```python
from build123d import *

# Parameters (mm, degrees)
ESQUISSE1_R             = 1.7
BOSS_EXTRU_1_DEPTH      = 3
ESQUISSE2_R             = 5.2
BOSS_EXTRU_2_DEPTH      = 3
BOSS_EXTRU_2_DEPTH_BACK = 3
ESQUISSE5_W             = 129.390100882
ESQUISSE5_H             = 125.631489025
ENL_V_MAT_EXTRU_2_DEPTH = 1
ESQUISSE6_R             = 1.5
ENL_V_MAT_EXTRU_3_DEPTH = 8
ESQUISSE7_W             = 14.610679854
ESQUISSE7_H             = 62.75
ENL_V_MAT_EXTRU_4_DEPTH = 8
BOSS_EXTRU_3_DEPTH      = 7
BOSS_EXTRU_4_DEPTH      = 7
ESQUISSE11_W            = 143.807333736
ESQUISSE11_H            = 19.954067826
ENL_V_MAT_EXTRU_5_DEPTH = 89
ESQUISSE12_R            = 1.7
ENL_V_MAT_EXTRU_6_DEPTH = 31


with BuildPart() as part:
    # Esquisse1 → Boss.-Extru.1 (new body)
    with BuildSketch(Plane.XY):
        with BuildLine():
            Line((-117.680084405, 66.939310237), (-117.680084405, 59.695120061))
            ThreePointArc((-117.680084405, 59.695120061), (-116.069171702, 55.806032765), (-112.180084405, 54.195120061))
            Line((-112.180084405, 54.195120061), (-105.294175096, 54.195120061))
            ThreePointArc((-105.294175096, 54.195120061), (-101.4050878, 52.584207358), (-99.794175096, 48.695120061))
            Line((-99.794175096, 48.695120061), (-99.794175096, 35.930823665))
            ThreePointArc((-99.794175096, 35.930823665), (-101.4050878, 32.041736368), (-105.294175096, 30.430823665))
            Line((-105.294175096, 30.430823665), (-112.180084405, 30.430823665))
            ThreePointArc((-112.180084405, 30.430823665), (-116.069171702, 28.819910961), (-117.680084405, 24.930823665))
            Line((-117.680084405, 24.930823665), (-117.680084405, 23.910007682))
            ThreePointArc((-117.680084405, 23.910007682), (-116.069171702, 20.020920385), (-112.180084405, 18.410007682))
            Line((-112.180084405, 18.410007682), (-105.294175096, 18.410007682))
            ThreePointArc((-105.294175096, 18.410007682), (-101.4050878, 16.799094979), (-99.794175096, 12.910007682))
            Line((-99.794175096, 12.910007682), (-99.794175096, 1.692208933))
            ThreePointArc((-99.794175096, 1.692208933), (-101.4050878, -2.196878364), (-105.294175096, -3.807791067))
            Line((-105.294175096, -3.807791067), (-113.390601299, -3.807791067))
            ThreePointArc((-113.390601299, -3.807791067), (-117.279688595, -5.418703771), (-118.890601299, -9.307791067))
            Line((-118.890601299, -9.307791067), (-118.890601299, -18.42196685))
            Line((-118.890601299, -18.42196685), (-118.890601299, -32.5606385))
            ThreePointArc((-118.890601299, -32.5606385), (-117.279688595, -36.449725797), (-113.390601299, -38.0606385))
            Line((-113.390601299, -38.0606385), (-52.866544484, -38.0606385))
            ThreePointArc((-52.866544484, -38.0606385), (-48.977457187, -36.449725797), (-47.366544484, -32.5606385))
            Line((-47.366544484, -32.5606385), (-47.366544484, -18.42196685))
            Line((-47.366544484, -18.42196685), (-47.366544484, -9.307791067))
            ThreePointArc((-47.366544484, -9.307791067), (-48.977457187, -5.418703771), (-52.866544484, -3.807791067))
            Line((-52.866544484, -3.807791067), (-77.986378892, -3.807791067))
            ThreePointArc((-77.986378892, -3.807791067), (-81.875466189, -2.196878364), (-83.486378892, 1.692208933))
            Line((-83.486378892, 1.692208933), (-83.486378892, 12.910007682))
            ThreePointArc((-83.486378892, 12.910007682), (-81.875466189, 16.799094979), (-77.986378892, 18.410007682))
            Line((-77.986378892, 18.410007682), (-69.856378892, 18.410007682))
            ThreePointArc((-69.856378892, 18.410007682), (-65.967291596, 20.020920385), (-64.356378892, 23.910007682))
            Line((-64.356378892, 23.910007682), (-64.356378892, 24.930823665))
            ThreePointArc((-64.356378892, 24.930823665), (-65.967291596, 28.819910961), (-69.856378892, 30.430823665))
            Line((-69.856378892, 30.430823665), (-77.986378892, 30.430823665))
            ThreePointArc((-77.986378892, 30.430823665), (-81.875466189, 32.041736368), (-83.486378892, 35.930823665))
            Line((-83.486378892, 35.930823665), (-83.486378892, 55.219310237))
            ThreePointArc((-83.486378892, 55.219310237), (-81.875466189, 59.108397534), (-77.986378892, 60.719310237))
            Line((-77.986378892, 60.719310237), (-54.190366806, 60.719310237))
            ThreePointArc((-54.190366806, 60.719310237), (-50.30127951, 62.330222941), (-48.690366806, 66.219310237))
            Line((-48.690366806, 66.219310237), (-48.690366806, 67.219310237))
            ThreePointArc((-48.690366806, 67.219310237), (-50.30127951, 71.108397534), (-54.190366806, 72.719310237))
            Line((-54.190366806, 72.719310237), (-112.180084405, 72.719310237))
            ThreePointArc((-112.180084405, 72.719310237), (-116.069171702, 71.108397534), (-117.680084405, 67.219310237))
            Line((-117.680084405, 67.219310237), (-117.680084405, 66.939310237))
        make_face()
        with Locations((-59.266378892, -15.663707737)):
            Circle(ESQUISSE1_R, mode=Mode.SUBTRACT)
        with Locations((-59.266378892, 66.939310237)):
            Circle(ESQUISSE1_R, mode=Mode.SUBTRACT)
        with Locations((-91.856378892, 36.719310237)):
            Circle(ESQUISSE1_R, mode=Mode.SUBTRACT)
        with Locations((-107.466378892, -14.520689763)):
            Circle(ESQUISSE1_R, mode=Mode.SUBTRACT)
        with Locations((-107.466378892, 60.719310237)):
            Circle(ESQUISSE1_R, mode=Mode.SUBTRACT)
        with Locations((-58.306378892, -31.603707737)):
            Circle(ESQUISSE1_R, mode=Mode.SUBTRACT)
        with Locations((-108.486378892, -31.600689763)):
            Circle(ESQUISSE1_R, mode=Mode.SUBTRACT)
        with BuildLine():
            Line((-111.390601299, 21.460065469), (-70.086378892, 21.460065469))
            ThreePointArc((-70.086378892, 21.460065469), (-68.67216533, 22.045851906), (-68.086378892, 23.460065469))
            Line((-68.086378892, 23.460065469), (-68.086378892, 24.842520386))
            ThreePointArc((-68.086378892, 24.842520386), (-68.67216533, 26.256733949), (-70.086378892, 26.842520386))
            Line((-70.086378892, 26.842520386), (-111.390601299, 26.842520386))
            ThreePointArc((-111.390601299, 26.842520386), (-112.804814861, 26.256733949), (-113.390601299, 24.842520386))
            Line((-113.390601299, 24.842520386), (-113.390601299, 23.460065469))
            ThreePointArc((-113.390601299, 23.460065469), (-112.804814861, 22.045851906), (-111.390601299, 21.460065469))
        make_face(mode=Mode.SUBTRACT)
    extrude(amount=BOSS_EXTRU_1_DEPTH)

    # Esquisse2 → Boss.-Extru.2 (add, two sides)
    with BuildSketch(Plane(origin=(0, 0, 0), x_dir=(-1, 0, 0), z_dir=(0, 0, -1))) as boss_extru_2_sk:
        with BuildLine():
            Line((118.890601299, -9.969506719), (130.584615963, -9.880075131))
            ThreePointArc((130.584615963, -9.880075131), (134.095405897, -8.402210456), (135.546378892, -4.880221341))
            Line((135.546378892, -4.880221341), (135.546378892, 5.415623015))
            ThreePointArc((135.546378892, 5.415623015), (136.425058549, 7.536943358), (138.546378892, 8.415623015))
            Line((138.546378892, 8.415623015), (145.752654566, 8.415623015))
            ThreePointArc((145.752654566, 8.415623015), (147.87397491, 9.294302671), (148.752654566, 11.415623015))
            Line((148.752654566, 11.415623015), (148.752654566, 38.179170847))
            ThreePointArc((148.752654566, 38.179170847), (147.87397491, 40.300491191), (145.752654566, 41.179170847))
            Line((145.752654566, 41.179170847), (138.546378892, 41.179170847))
            ThreePointArc((138.546378892, 41.179170847), (136.425058549, 42.057850504), (135.546378892, 44.179170847))
            Line((135.546378892, 44.179170847), (135.546378892, 52.099902349))
            ThreePointArc((135.546378892, 52.099902349), (134.081912798, 55.635436255), (130.546378892, 57.099902349))
            Line((130.546378892, 57.099902349), (117.680084405, 57.099902349))
            Line((117.680084405, 57.099902349), (117.680084405, 72.719310237))
            Line((117.680084405, 72.719310237), (48.690366806, 72.719310237))
            Line((48.690366806, 72.719310237), (48.690366806, 60.719310237))
            Line((48.690366806, 60.719310237), (48.690366806, 57.099902349))
            Line((48.690366806, 57.099902349), (40.256901013, 57.099902349))
            ThreePointArc((40.256901013, 57.099902349), (37.428473888, 55.928329474), (36.256901013, 53.099902349))
            Line((36.256901013, 53.099902349), (36.256901013, 47.456292263))
            Line((36.256901013, 47.456292263), (39.346378892, 47.456292263))
            ThreePointArc((39.346378892, 47.456292263), (41.396631424, 52.406039732), (46.346378892, 54.456292263))
            Line((46.346378892, 54.456292263), (126.246378892, 54.456292263))
            ThreePointArc((126.246378892, 54.456292263), (131.196126361, 52.406039732), (133.246378892, 47.456292263))
            Line((133.246378892, 47.456292263), (133.246378892, 40.977229779))
            ThreePointArc((133.246378892, 40.977229779), (134.125058549, 38.855909436), (136.246378892, 37.977229779))
            Line((136.246378892, 37.977229779), (142.162261637, 37.977229779))
            ThreePointArc((142.162261637, 37.977229779), (144.28358198, 37.098550123), (145.162261637, 34.977229779))
            Line((145.162261637, 34.977229779), (145.162261637, 14.363062522))
            ThreePointArc((145.162261637, 14.363062522), (144.28358198, 12.241742179), (142.162261637, 11.363062522))
            Line((142.162261637, 11.363062522), (136.246378892, 11.363062522))
            ThreePointArc((136.246378892, 11.363062522), (134.125058549, 10.484382866), (133.246378892, 8.363062522))
            Line((133.246378892, 8.363062522), (133.246378892, -1.293707737))
            ThreePointArc((133.246378892, -1.293707737), (131.196126361, -6.243455205), (126.246378892, -8.293707737))
            Line((126.246378892, -8.293707737), (46.346378892, -8.293707737))
            ThreePointArc((46.346378892, -8.293707737), (41.396631424, -6.243455205), (39.346378892, -1.293707737))
            Line((39.346378892, -1.293707737), (36.248203357, -1.293707737))
            Line((36.248203357, -1.293707737), (36.248203357, -6.64542392))
            ThreePointArc((36.248203357, -6.64542392), (37.432020164, -9.486042202), (40.282759469, -10.645274652))
            Line((40.282759469, -10.645274652), (47.366544484, -10.58407535))
            Line((47.366544484, -10.58407535), (47.366544484, -23.92196685))
            Line((47.366544484, -23.92196685), (118.890601299, -23.92196685))
            Line((118.890601299, -23.92196685), (118.890601299, -9.969506719))
        make_face()
        with Locations((59.266378892, -15.663707737)):
            Circle(ESQUISSE2_R, mode=Mode.SUBTRACT)
        with Locations((107.466378892, -14.520689763)):
            Circle(ESQUISSE2_R, mode=Mode.SUBTRACT)
        with Locations((107.466378892, 60.719310237)):
            Circle(ESQUISSE2_R, mode=Mode.SUBTRACT)
        with Locations((59.266378892, 66.939310237)):
            Circle(ESQUISSE2_R, mode=Mode.SUBTRACT)
    extrude(amount=BOSS_EXTRU_2_DEPTH)
    extrude(boss_extru_2_sk.sketch, amount=-BOSS_EXTRU_2_DEPTH_BACK)

    # Esquisse5 → Enl_v. mat.-Extru.2 (cut)
    with BuildSketch(Plane.XY.offset(3)):
        with Locations((-91.695706627, 17.054727605)):
            Rectangle(ESQUISSE5_W, ESQUISSE5_H)
    extrude(amount=-ENL_V_MAT_EXTRU_2_DEPTH, mode=Mode.SUBTRACT)

    # Esquisse6 → Enl_v. mat.-Extru.3 (cut)
    with BuildSketch(Plane.XY.offset(2)):
        with Locations((-69.623492164, 64.727424081)):
            Circle(ESQUISSE6_R)
        with Locations((-83.623492164, 64.727424081)):
            Circle(ESQUISSE6_R)
    extrude(amount=-ENL_V_MAT_EXTRU_3_DEPTH, mode=Mode.SUBTRACT)

    # Esquisse7 → Enl_v. mat.-Extru.4 (cut)
    with BuildSketch(Plane(origin=(0, 0, 0), x_dir=(-1, 0, 0), z_dir=(0, 0, -1))):
        with Locations((42.567758063, 23.081292263)):
            Rectangle(ESQUISSE7_W, ESQUISSE7_H)
    extrude(amount=ENL_V_MAT_EXTRU_4_DEPTH, mode=Mode.SUBTRACT)

    # Esquisse9 → Boss.-Extru.3 (add)
    with BuildSketch(Plane(origin=(0, -1.293707737, 0), x_dir=(1, 0, 0), z_dir=(0, 1, 0))):
        Polygon((-39.346378892, -2), (-39.346378892, 0.886005049), (-36.248203357, 0), (-36.248203357, -2), align=None)
    extrude(amount=-BOSS_EXTRU_3_DEPTH)

    # Esquisse10 → Boss.-Extru.4 (add)
    with BuildSketch(Plane.XZ.offset(-47.456292263)):
        Polygon((-39.346378892, 2), (-39.346378892, -0.873043126), (-36.256901013, 0), (-36.256901013, 2), align=None)
    extrude(amount=-BOSS_EXTRU_4_DEPTH)

    # Esquisse11 → Enl_v. mat.-Extru.5 (cut)
    with BuildSketch(Plane(origin=(0, -1.293707737, 0), x_dir=(1, 0, 0), z_dir=(0, 1, 0))):
        with Locations((-95.995427174, 3.905261548)):
            Rectangle(ESQUISSE11_W, ESQUISSE11_H)
    extrude(amount=ENL_V_MAT_EXTRU_5_DEPTH, mode=Mode.SUBTRACT)

    # Esquisse12 → Enl_v. mat.-Extru.6 (cut)
    with BuildSketch(Plane.XY.offset(2)):
        with Locations((-103.175863959, -31.601009153)):
            Circle(ESQUISSE12_R)
        with Locations((-87.885863987, -31.601928739)):
            Circle(ESQUISSE12_R)
        with Locations((-80.977833602, -31.748759482)):
            Circle(ESQUISSE12_R)
        with Locations((-61.977833602, -31.748759482)):
            Circle(ESQUISSE12_R)
    extrude(amount=-ENL_V_MAT_EXTRU_6_DEPTH, mode=Mode.SUBTRACT)


solid = part.part
```
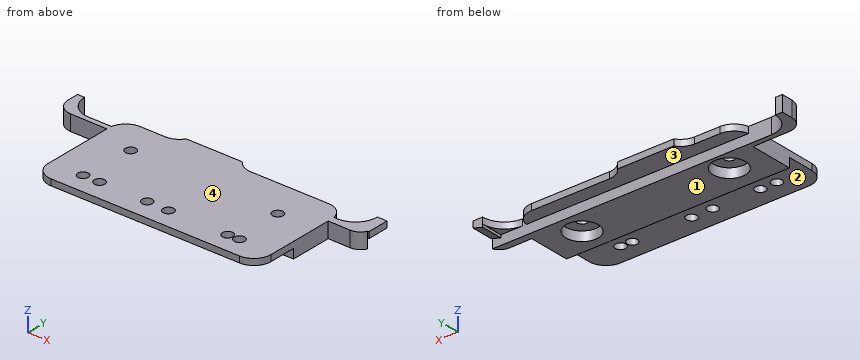
Verification items for the finished model (mm, model axes). Face numbers are marked on the shaded views. A direction names the side the tool comes from. Give positions to 0.01 mm unless a question says otherwise; leave off trailing zeros. Order: outer loops, then holes, each group sorted by start corner. A loop starts at its lowest first (then second) coordinate and runs counter-clockwise, first axis right, second up. Notation, with made-up numbers: (67.5, 38) -> (123.5, 38) arc R13 cw to (123.5, 55) -> close; hole circle Ø6 at (73, -21.75). An arc over 180 degrees is marked (long way). Use a Markdown table: item, result.
1) Section check C-C, the plane y = -27. Record the boundary of the cut face in (x, z), then the cut area to 3 significant figures.
Results:
| item | result |
|---|---|
| outline | (-118.89, 0) -> (-47.37, 0) -> (-47.37, 2) -> (-118.89, 2) -> close |
| area | 143 mm² |
2) Section check D-D, the plane y = -34.5. Record the boundary of the cut face in (x, z), then the cut area to 3 significant figures.
Results:
| item | result |
|---|---|
| outline | (-118.54, 0) -> (-47.72, 0) -> (-47.72, 2) -> (-118.54, 2) -> close |
| area | 142 mm² |
3) Section check B-B, the plane x = -84. Record the boundary of the cut face in (y, z), then the cut area to 3 significant figures.
Results:
| item | result |
|---|---|
| outline | (-38.06, 0) -> (-23.92, 0) -> (-23.92, -3) -> (-8.29, -3) -> (-8.29, 0) -> (-1.29, 0) -> (-1.29, 2) -> (-38.06, 2) -> close |
| area | 120 mm² |
4) Depth check by flat-ended pin: pin 1 Ø2.5 at (x, y) = (-58.31, -31.6) entering from +Z; pin 2 Ø1.5 at (x, z) = (-61, 1.5) entering from +Y; pin 3 Ø9.5 at (x, y) = (-59.27, -15.66) entering from -Z; pin 4 Ø1.5 at (x, z) = (-80, -1) entering from +Y. Enter the tip coordinate at first touch or a pass-through.
Results:
| item | result |
|---|---|
| pin 1 | through |
| pin 2 | y = -3.81 |
| pin 3 | z = 0 |
| pin 4 | y = -8.29 |
5) Section check A-A, the plane x = -62.5. Record the boundary of the cut face in (y, z), then the cut area to 3 significant figures.
Results:
| item | result |
|---|---|
| outline | (-38.06, 0) -> (-33.37, 0) -> (-33.37, 2) -> (-38.06, 2) -> close; (-30.13, 0) -> (-23.92, 0) -> (-23.92, -3) -> (-19.74, -3) -> (-19.74, 0) -> (-11.59, 0) -> (-11.59, -3) -> (-8.29, -3) -> (-8.29, 0) -> (-3.81, 0) -> (-3.81, 2) -> (-30.13, 2) -> close |
| area | 84.5 mm² |
6) Tool access check on the marked faces 1 and 2. Record the directions out of +Z, -Z, +X, -X, +Y, -Y that give a thin tool (end or side, any length) a straight path to the whole face; none if there is none.
Results:
| item | result |
|---|---|
| face 1 | -Z, +X, -X, +Y, -Y |
| face 2 | -Z, +X, -X, -Y |
7) Mould release check, pull along X, two halves, no side actions. Record for the marked faces 3 and 4: pulls with the +X half, pulls with the -X half, needs draft (parallel to the pull), parting line crosses it, or undercut.
Results:
| item | result |
|---|---|
| face 3 | undercut |
| face 4 | needs draft |
8) Material ranges on probe 1 along X at (y, z) = (-15.5, -0.25); probe 2 along Z at (x, y) = (-88.5, -2.5); probe 3 along X at (y, z) = (-14, -1.7), recorded low to high.
Results:
| item | result |
|---|---|
| probe 1 | -118.89 to -112.57, -102.36 to -64.46, -54.07 to -47.37 |
| probe 2 | 0 to 2 |
| probe 3 | -118.89 to -112.64, -102.29 to -64.19, -54.34 to -47.37 |
